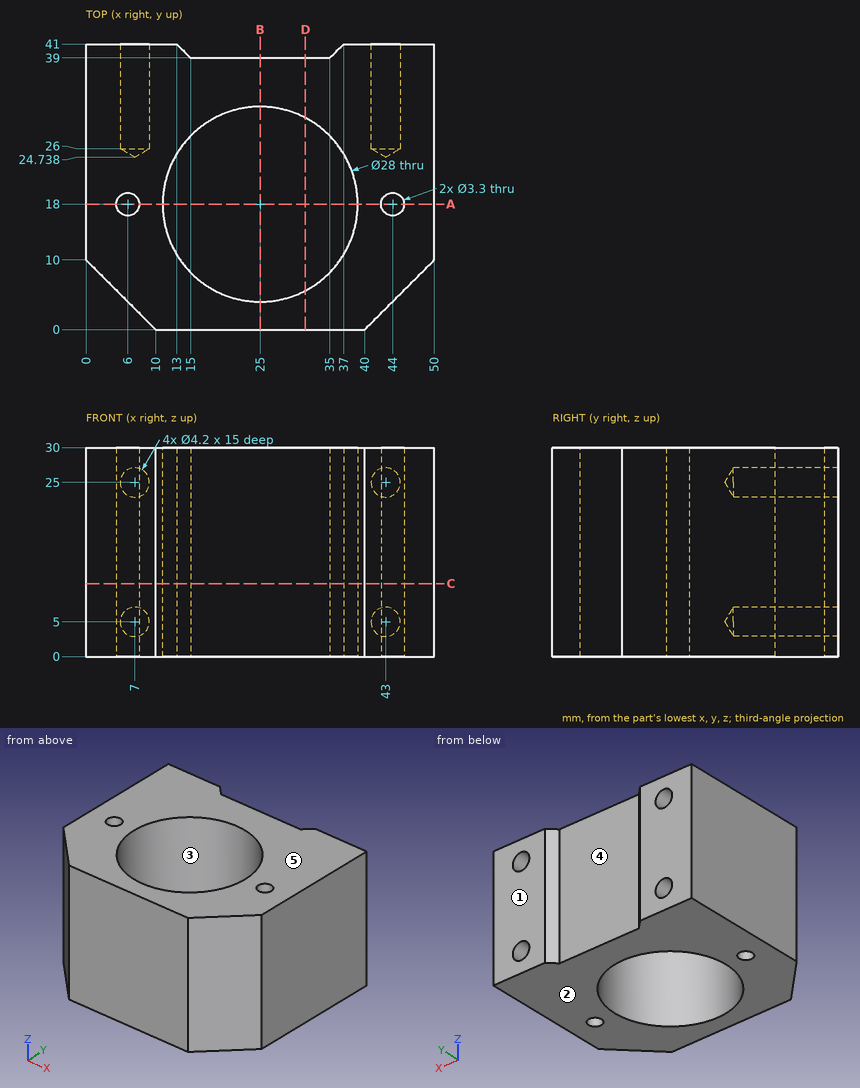
Drawing for the job (mm, zero at the part's lowest x, y, z). A direction names the side the tool comes from. Round coordinates to 2 decimals unless told otherwise and drop trailing zeros. Loops run counter-clockwise (first coordinate to the right, second up) from the corner with the lowest first, then second, coordinate; pieces in that order, holes last.
1. Band-saw the part on C-C, the plane z = 10.5. Count the separate pieces of the cut face and the enclosed holes in it, and give its area (3 significant figures).
Check values:
separate pieces: 1
enclosed holes: 3
area: 1,270 mm2
2. Wall check: probe 1 along Z at (x, y) = (43, 35); probe 2 along Y at (x, z) = (6, 19); probe 3 along Y at (x, z) = (25, 23). Give the ranges that are in metal, low to high.
Check values:
probe 1: z = 0 to 2.9, 7.1 to 22.9, 27.1 to 30
probe 2: y = 4 to 16.35, 19.65 to 41
probe 3: y = 0 to 4, 32 to 39
3. Tool access for the marked faces 4 and 5: list every direction of +Z, -Z, +X, -X, +Y, -Y with a clear straight run to the whole face (end or side of a thin tool).
Check values:
face 4: +Z, -Z, +Y
face 5: +Z, +X, -X, +Y, -Y
4. Band-saw the part on D-D, the plane x = 31.5. List the corners of the cut face in (y, z).
Check values:
outline: (0, 0) - (5.6, 0) - (5.6, 30) - (0, 30) - close; (30.4, 0) - (39, 0) - (39, 30) - (30.4, 30) - close
5. Band-saw the part on A-A, the plane y = 18. List the corners of the cut face in (x, z), and give its area (3 significant figures).
Check values:
outline: (0, 0) - (4.35, 0) - (4.35, 30) - (0, 30) - close; (7.65, 0) - (11, 0) - (11, 30) - (7.65, 30) - close; (39, 0) - (42.35, 0) - (42.35, 30) - (39, 30) - close; (45.65, 0) - (50, 0) - (50, 30) - (45.65, 30) - close
area: 462 mm2
6. Band-saw the part on B-B, the plane x = 25. List the corners of the cut face in (y, z).
Check values:
outline: (0, 0) - (4, 0) - (4, 30) - (0, 30) - close; (32, 0) - (39, 0) - (39, 30) - (32, 30) - close
7. Mould opens along Y. For the marked faces 1, 2 and 3 say: +Y half, -Y half, draft (parallel to the pull), parting line (faces both ways), or undercut.
Check values:
face 1: +Y half
face 2: draft
face 3: undercut
8. Drop flat-ended pins along their axis: P1, Ø5.5, axis at x = 43, z = 25, coming from the -Y side; P2, Ø3.5, axis at x = 7, z = 5, coming from the +Y side; P3, Ø10, axis at x = 27, z = 9, coming from the +Y side. Give the stop position or say it passes through.
Check values:
P1: stops at y = 0.25
P2: stops at y = 25.79
P3: stops at y = 39
